from build123d import *

# Parameters (mm, degrees)
F1_DEPTH = 1.5


with BuildPart() as f1:
    # F0 (on Front) → F1 (new body)
    with BuildSketch(Plane.XZ):
        with BuildLine():
            Line((0, -12), (0, -6))
            Line((0, -6), (10.392305, -6))
            ThreePointArc((10.392305, -6), (11.59111, -3.105829), (12, 0))
            ThreePointArc((12, 0), (-8.485281, 8.485281), (0, -12))
        make_face()
        with BuildLine():
            ThreePointArc((0, -6), (-4.242641, 4.242641), (6, 0))
            ThreePointArc((6, 0), (4.242641, -4.242641), (0, -6))
        make_face(mode=Mode.SUBTRACT)
        with BuildLine():
            Line((18, -6), (10.392305, -6))
            ThreePointArc((10.392305, -6), (6, -10.392305), (0, -12))
            Line((0, -12), (18, -12))
            Line((18, -12), (18, -6))
        make_face()
        with BuildLine():
            Line((10.392305, -6), (0, -6))
            Line((0, -6), (0, -12))
            ThreePointArc((0, -12), (6, -10.392305), (10.392305, -6))
        make_face()
    extrude(amount=F1_DEPTH)


solid = f1.part
Build history of the part. All positions in model axes, mm. Give positions to 0.01 mm unless a question says otherwise; leave off trailing zeros. Order: outer loops, then holes, each group sorted by start corner. A loop starts at its lowest first (then second) coordinate and runs counter-clockwise, first axis right, second up. Notation, with made-up numbers: M 81,84.25 L 121,84.25 A27 ccw 121,118.25 Z; hole C 21,-23.75 d3. An arc over 180 degrees is marked long. Use one line per item in the form item = value.
1) Saw through at C-C (x = 14). Give the cut face in (y, z).
Calculated:
outline = M -1.5,-12 L 0,-12 L 0,-6 L -1.5,-6 Z
2) Saw through at B-B (z = 5). Give the cut face in (x, y), plus the area to 3 significant figures.
Calculated:
outline = M -10.91,-1.5 L -3.32,-1.5 L -3.32,0 L -10.91,0 Z; M 3.32,-1.5 L 10.91,-1.5 L 10.91,0 L 3.32,0 Z
area = 22.8 mm2
3) Saw through at A-A (y = -0.35). Give the cut face in (x, z), plus the area to 3 significant figures.
Calculated:
outline = M 0,-12 L 18,-12 L 18,-6 L 10.39,-6 A12 ccw 12,0 A12 ccw long Z; hole M 0,-6 A6 ccw 6,0 A6 ccw long Z
area = 403 mm2
4) Drop a flat-ended pin along its axis: pin 1 (0.8 mm diameter, centred on x = 14.5, y = -1, fed in from +Z). Give the stop position or say it passes through.
Calculated:
pin_1 = -6
5) Saw through at D-D (z = -2.5). Give the cut face in (x, y), plus the area to 3 significant figures.
Calculated:
outline = M -11.74,-1.5 L -5.45,-1.5 L -5.45,0 L -11.74,0 Z; M 5.45,-1.5 L 11.74,-1.5 L 11.74,0 L 5.45,0 Z
area = 18.8 mm2
6) Two-plate mould, pull along Z, no slides. Class faces 1 (the face through (6, 0, -2)), 2 (the face through (14, -1, -6)), 3 (the face through (9, -1, -12)): released by +Z, released by -Z, zero draft, split by the parting line, or undercut.
Calculated:
face_1 = zero draft
face_2 = undercut
face_3 = released by -Z
7) Probe probe 1 along Z at (x, y) = (14.25, -1.2); probe 2 along X at (y, z) = (-0.6, 2); probe 3 along Z at (x, y) = (2.75, -0.2). List the from-to ranges inside material, lowest first.
Calculated:
probe_1 = -12 to -6
probe_2 = -11.83 to -5.66, 5.66 to 11.83
probe_3 = -12 to -5.33, 5.33 to 11.68
